from build123d import *

# Parameters (mm, degrees)
SKETCH_1_W          = 100
SKETCH_1_H          = 5
EXTRUDE_1_DEPTH     = 8
SKETCH_2_R          = 1.1
CUT_EXTRUDE_1_DEPTH = 51.882216933
SKETCH_2_3_R        = 2
CUT_EXTRUDE_2_DEPTH = 3
CUT_EXTRUDE_3_DEPTH = 51.882216933
CUT_EXTRUDE_4_DEPTH = 51.882216933
EXTRUDE_START       = 20
SKETCH_4_W          = 15
SKETCH_4_H          = 8
EXTRUDE_2_DEPTH     = 20
CUT_EXTRUDE_5_DEPTH = 56.409836672


with BuildPart() as part:
    # 草图1 → 凸台-拉伸1 (new body)
    with BuildSketch(Plane(origin=(0, 0, 0), x_dir=(1, 0, 0), z_dir=(0, 1, 0))):
        Rectangle(SKETCH_1_W, SKETCH_1_H)
    extrude(amount=EXTRUDE_1_DEPTH)

    # 草图2 → 切除-拉伸1 (cut, through all)
    with BuildSketch(Plane.XY.offset(2.5)):
        with Locations((46, 4)):
            Circle(SKETCH_2_R)
        with Locations((36, 4)):
            Circle(SKETCH_2_R)
    extrude(amount=-CUT_EXTRUDE_1_DEPTH, mode=Mode.SUBTRACT)

    # 草图2<3> → 切除-拉伸2 (cut)
    with BuildSketch(Plane.XY.offset(2.5)):
        with Locations((36, 4)):
            Circle(SKETCH_2_3_R)
        with Locations((46, 4)):
            Circle(SKETCH_2_3_R)
    extrude(amount=-CUT_EXTRUDE_2_DEPTH, mode=Mode.SUBTRACT)

    # 草图3 → 切除-拉伸3 (cut, through all)
    with BuildSketch(Plane.XY.offset(2.5)):
        with BuildLine():
            ThreePointArc((50, 4), (48.828427125, 1.171572875), (46, 0))
            Line((46, 0), (50, 0))
            Line((50, 0), (50, 4))
        make_face()
        with BuildLine():
            Line((50, 8), (46, 8))
            ThreePointArc((46, 8), (48.828427125, 6.828427125), (50, 4))
            Line((50, 4), (50, 8))
        make_face()
    extrude(amount=-CUT_EXTRUDE_3_DEPTH, mode=Mode.SUBTRACT)

    # 草图3<3> → 切除-拉伸4 (cut, through all)
    with BuildSketch(Plane.XY.offset(2.5)):
        with BuildLine():
            ThreePointArc((-50, 4), (-48.828427125, 6.828427125), (-46, 8))
            Line((-46, 8), (-50, 8))
            Line((-50, 8), (-50, 4))
        make_face()
        with BuildLine():
            Line((-50, 0), (-46, 0))
            ThreePointArc((-46, 0), (-48.828427125, 1.171572875), (-50, 4))
            Line((-50, 4), (-50, 0))
        make_face()
    extrude(amount=-CUT_EXTRUDE_4_DEPTH, mode=Mode.SUBTRACT)

    # 草图4 → 凸台-拉伸2 (add)
    with BuildSketch(Plane.XY.offset(2.5).offset(EXTRUDE_START)):
        with BuildLine():
            Line((-46, 0), (-46, 8))
            ThreePointArc((-46, 8), (-50, 4), (-46, 0))
        make_face()
        with Locations((-38.5, 4)):
            Rectangle(SKETCH_4_W, SKETCH_4_H)
    extrude(amount=-EXTRUDE_2_DEPTH)

    # 草图5 → 切除-拉伸5 (cut, through all)
    with BuildSketch(Plane.XZ):
        with BuildLine():
            ThreePointArc((-33.5, 12.5), (-38.5, 17.5), (-43.5, 12.5))
            Line((-43.5, 12.5), (-33.5, 12.5))
        make_face()
        with BuildLine():
            Line((-33.5, 12.5), (-43.5, 12.5))
            ThreePointArc((-43.5, 12.5), (-38.5, 7.5), (-33.5, 12.5))
        make_face()
    extrude(amount=-CUT_EXTRUDE_5_DEPTH, mode=Mode.SUBTRACT)


solid = part.part
Can you work these out from the model? Positions are in its coordinate system, mm. A direction names the side the tool comes from. Give positions to 0.01 mm unless a question says otherwise; leave off trailing zeros. Order: outer loops, then holes, each group sorted by start corner. A loop starts at its lowest first (then second) coordinate and runs counter-clockwise, first axis right, second up. Notation, with made-up numbers: M -11,38 L 9,38 A36 ccw 9,75 Z; hole C 9.25,-39.5 d2. An arc over 180 degrees is marked long. Use one line per item in the form item = value. Start each with the question number.
Item 1: If I drill on line 1 along Y through (x, z) = (36, -1.05); line 2 along X through (y, z) = (3, 0); line 3 along Z through (x, y) = (-14, 3), over which ranges is the centre line in solid material (lowest first)?
Item 2: If we section it at A-A (z = 1.5): Write out the boundary of the cut face in (x, y), then the cut area to 3 significant figures.
Item 3: Will these pins go through, and if not, where does the flat tip stop? pin 1 Ø4.5 at (x, y) = (45.5, 3.5) entering from +Z; pin 2 Ø1.5 at (y, z) = (2, 10.5) entering from -X.
Item 4: If we section it at C-C (y = 1): Write out the boundary of the cut face in (x, z).
Item 5: If we section it at D-D (z = 11.25): Write out the boundary of the cut face in (x, y).
Item 6: We'd pull the mould along X, two halves only. Please class faces 1 (the flat face through (-1, 4, -2.5)), 2 (the flat face through (-31, 4, 13)), 3 (the cylindrical face through (-33.505, 3.944, 12.28)): +X half, -X half, draft (parallel to the pull), parting line (faces both ways), or undercut.
Item 7: If we section it at B-B (x = 36): Write out the boundary of the cut face in (y, z), then the cut area to 3 significant figures.
Item 8: For faces 4 (the flat face through (-41, 4, 22.5)), 5 (the cylindrical face through (47.847, 3.234, 1.021)), 6 (the flat face through (9, 4, 2.5)), which set-ups out of +Z, -Z, +X, -X, +Y, -Y let a thin tool reach every point of the face, with its end or its side?
Outcome:
q1.line_1 = 0 to 2.9, 5.1 to 8
q1.line_2 = -49.87 to 34.27, 37.73 to 44.27, 47.73 to 49.87
q1.line_3 = -2.5 to 2.5
q2.outline = M -46,0 L 46,0 A4 ccw 46,8 L -46,8 A4 ccw Z; hole C 36,4 d4; hole C 46,4 d4
q2.area = 761 mm2
q3.pin_1 = 2.5
q3.pin_2 = -49.8
q4.outline = M -48.65,-2.5 L 48.65,-2.5 L 48.65,2.5 L -31,2.5 L -31,22.5 L -48.65,22.5 Z; hole C -38.5,12.5 d10
q5.outline = M -46,0 L -43.34,0 L -43.34,8 L -46,8 A4 ccw Z; M -33.66,0 L -31,0 L -31,8 L -33.66,8 Z
q6.face_1 = draft
q6.face_2 = +X half
q6.face_3 = undercut
q7.outline = M 0,-2.5 L 2.9,-2.5 L 2.9,-0.5 L 2,-0.5 L 2,2.5 L 0,2.5 Z; M 5.1,-2.5 L 8,-2.5 L 8,2.5 L 6,2.5 L 6,-0.5 L 5.1,-0.5 Z
q7.area = 23.6 mm2
q8.face_4 = +Z, +X, -X, +Y, -Y
q8.face_5 = +Z
q8.face_6 = +Z, +X, +Y, -Y
